Input: part model. Units: mm. Frame: model coordinates. Give positions to 0.01 mm unless a question says otherwise; leave off trailing zeros. Loops run counter-clockwise (first coordinate to the right, second up) from the corner with the lowest first, then second, coordinate; pieces in that order, holes last. Notation, with made-up numbers: M -13,-38.5 L 10,-38.5 A34 cw 10,-4.5 Z; hole C 77.5,4 d11. An arc over 180 degrees is marked long. Use CSV: the item, a comma, the result in double quotes. Start each with the question number.
Q1. Section A-A, the plane y = 0.5. Output: boundary loops of the cut face in (x, z), plus the area to 3 significant figures.
Q2. Section B-B, the plane x = 2. Output: boundary loops of the cut face in (y, z), plus the area to 3 significant figures.
Q3. Material intervals for line 1 along Z through (x, y) = (1.5, 0); line 2 along Z through (x, y) = (8.8, 0); line 3 along Z through (x, y) = (3.75, 5.5), sorted ascending.
Q4. Pin query (flat end, axial travel): pin 1 (3 mm diameter, centred on y = -1, z = 10, fed in from -X). Return the tip coordinate at first contact, or that it passes through.
Q5. Section C-C, the plane y = 12.5. Output: boundary loops of the cut face in (x, z), plus the area to 3 significant figures.
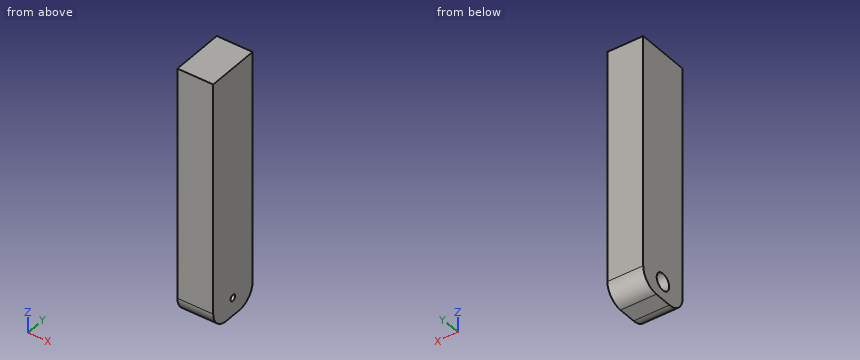
from build123d import *

# Parameters (mm, degrees)
SKETCH1_W           = 20
SKETCH1_H           = 30
BOSS_EXTRUDE1_DEPTH = 140
FILLET1_R           = 10
SKETCH2_R           = 1.75
CUT_EXTRUDE1_DEPTH  = 143.214626533
SKETCH3_R           = 4.75
CUT_EXTRUDE2_DEPTH  = 15


with BuildPart() as part:
    # Sketch1 → Boss-Extrude1 (new body)
    with BuildSketch(Plane.XY):
        Rectangle(SKETCH1_W, SKETCH1_H)
    extrude(amount=BOSS_EXTRUDE1_DEPTH)

    # Fillet1
    fillet1_edges = [part.edges().sort_by_distance(p)[0] for p in [
        (0, -15, 0),
        (0, 15, 0),
    ]]
    fillet(fillet1_edges, radius=FILLET1_R)

    # Sketch2 → Cut-Extrude1 (cut, through all)
    with BuildSketch(Plane(origin=(10, 0, 0), x_dir=(0, 0, -1), z_dir=(1, 0, 0))):
        with Locations(Location((-10, 0, 0), (0, 0, 90))):
            Circle(SKETCH2_R)
    extrude(amount=-CUT_EXTRUDE1_DEPTH, mode=Mode.SUBTRACT)

    # Sketch3 → Cut-Extrude2 (cut)
    with BuildSketch(Plane.ZY.offset(10)):
        with Locations(Location((10, 0, 0), (0, 0, 270))):
            Circle(SKETCH3_R)
    extrude(amount=-CUT_EXTRUDE2_DEPTH, mode=Mode.SUBTRACT)


solid = part.part
A:
1,outline,"M -10,0 L 10,0 L 10,8.32 L 5,8.32 L 5,5.28 L -10,5.28 Z; M -10,14.72 L 5,14.72 L 5,11.68 L 10,11.68 L 10,140 L -10,140 Z"
1,area,"2,640 mm^2"
2,outline,"M -15,10 A10 ccw -5,0 L 5,0 A10 ccw 15,10 L 15,140 L -15,140 Z; hole C 0,10 d9.5"
2,area,"4,090 mm^2"
3,line 1,"0 to 5.25, 14.75 to 140"
3,line 2,"0 to 8.25, 11.75 to 140"
3,line 3,"0.01 to 140"
4,pin 1,"x = 5"
5,outline,"M -10,3.39 L 10,3.39 L 10,140 L -10,140 Z"
5,area,"2,730 mm^2"
